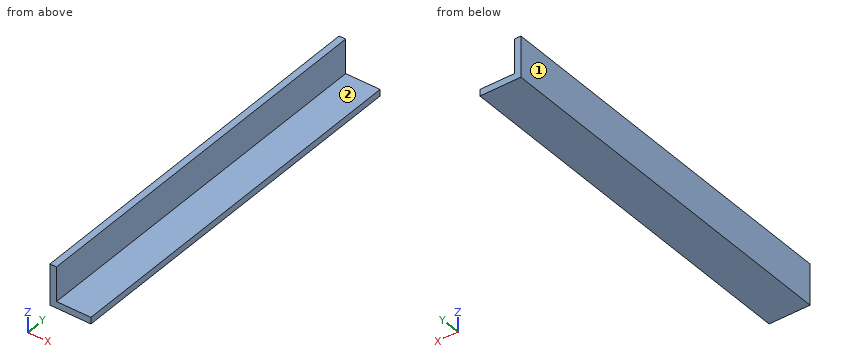
```python
from build123d import *

# Parameters (mm, degrees)
F0_W     = 9.53
F0_H     = 9.53
F1_DEPTH = 88
F2_T     = -1.53
F3_W     = 8
F3_H     = 1.53
F4_DEPTH = 88.001


with BuildPart() as f1:
    # F0 (on Front) → F1 (new body)
    with BuildSketch(Plane.XZ):
        with Locations((4.765, 4.765)):
            Rectangle(F0_W, F0_H)
    extrude(amount=F1_DEPTH)

    # F2
    f2_openings = [f1.faces().sort_by_distance(p)[0] for p in [
        (9.53, -44, 4.765),
        (4.765, -88, 4.765),
        (4.765, 0, 4.765),
    ]]
    offset(amount=F2_T, openings=f2_openings)

    # F3 (on Front) → F4 (cut, through all)
    with BuildSketch(Plane.XZ):
        with Locations((5.53, 8.765)):
            Rectangle(F3_W, F3_H)
    extrude(amount=F4_DEPTH, mode=Mode.SUBTRACT)


solid = f1.part
```
The model under review builds one solid part; all positions refer to its coordinate system, in mm. Face numbers are marked on the shaded views. A direction names the side the tool comes from. Round coordinates to 2 decimals unless told otherwise and drop trailing zeros. Loops run counter-clockwise (first coordinate to the right, second up) from the corner with the lowest first, then second, coordinate; pieces in that order, holes last. Notation, with made-up numbers: M 84,63 L 118,63 A15 cw 118,78 Z; hole C -35,60 d1. An arc over 180 degrees is marked long. Put each result on its own line as item: value.
Q1. For pin 1 (2 mm diameter, centred on y = -74.5, z = 4, fed in from +X); pin 2 (3 mm diameter, centred on x = 7.5, y = -67, fed in from +Z), all flat-tipped, find the tip position at first contact; note any pin that passes through.
Result set:
pin 1: stops at x = 1.53
pin 2: stops at z = 1.53
Q2. To check wall thickness, follow L1, parallel to X at y = -20, z = 3.5. State the ranges of the line that lie inside material, in increasing order.
Result set:
L1: x = 0 to 1.53
Q3. Consider section B-B, the plane z = 3.25. Give the boundary of the cut face in (x, y).
Result set:
outline: M 0,-88 L 1.53,-88 L 1.53,0 L 0,0 Z
Q4. Machinability: for the marked faces 1 and 2, which of the approach directions +Z, -Z, +X, -X, +Y, -Y give a long, thin tool a straight path to every point of the face, cutting with its end or side? Answer none if there is none.
Result set:
face 1: +Z, -Z, -X, +Y, -Y
face 2: +Z, +X, +Y, -Y
Q5. Consider section A-A, the plane y = -45.5. Give the boundary of the cut face in (x, z), then the cut area to 3 significant figures.
Result set:
outline: M 0,0 L 9.53,0 L 9.53,1.53 L 1.53,1.53 L 1.53,9.53 L 0,9.53 Z
area: 26.8 mm²
Q6. Consider section C-C, the plane x = 6.75. Give the boundary of the cut face in (y, z), then the cut area to 3 significant figures.
Result set:
outline: M -88,0 L 0,0 L 0,1.53 L -88,1.53 Z
area: 135 mm²
